Check sheet for the drawn part. Datum: minimum x, y, z corner. Units: mm. A direction names the side the tool comes from. Give positions to 0.01 mm unless a question says otherwise; leave off trailing zeros. Loops run counter-clockwise (first coordinate to the right, second up) from the corner with the lowest first, then second, coordinate; pieces in that order, holes last. Notation, with made-up numbers: (64.25, -12.5) - (89.25, -12.5) arc R10 ccw to (89.25, 2.5) - close; hole circle Ø5 at (-14, 44). An arc over 180 degrees is marked (long way). One line per item, written item: value. Start each with the question number.
1. Scan lines: L1, parallel to X at y = 3.9, z = 4; L2, parallel to Y at x = 10.75, z = 7; L3, parallel to Z at x = 8.75, y = 2.1. Record each from-to range of solid material in increasing order. Write a range as [from, to].
2. Sectioned sample at D-D (y = 1.65). Record the cut outline in (x, z), plus the area to 3 significant figures.
3. Sectioned sample at B-B (x = 7). Record the cut outline in (y, z), plus the area to 3 significant figures.
4. Sectioned sample at C-C (z = 4). Record the cut outline in (x, y).
5. Access from +Z, -Z, +X, -X, +Y, -Y to the whole of each face (thin tool, end or side, straight path). Record for the marked faces 1, 2, 3, 4 and 5.
6. Mould release check, pull along X, two halves, no side actions. Record for the marked faces 6, 7, 8 and 9: pulls with the +X half, pulls with the -X half, needs draft (parallel to the pull), parting line crosses it, or undercut.
7. Sectioned sample at A-A (y = 3). Record the cut outline in (x, z).
8. Gauge pin test, flat ends, axial feed: pin 1 (0.8 mm diameter, centred on y = 1.5, z = 4.5, fed in from -X); pin 2 (2 mm diameter, centred on x = 7, z = 4.5, fed in from +Y); pin 3 (2 mm diameter, centred on x = 6.5, y = 1, fed in from -Z); pin 4 (1 mm diameter, centred on y = 2.5, z = 2.5, fed in from -X). Record the tip position at first contact, or that the pin passes through.
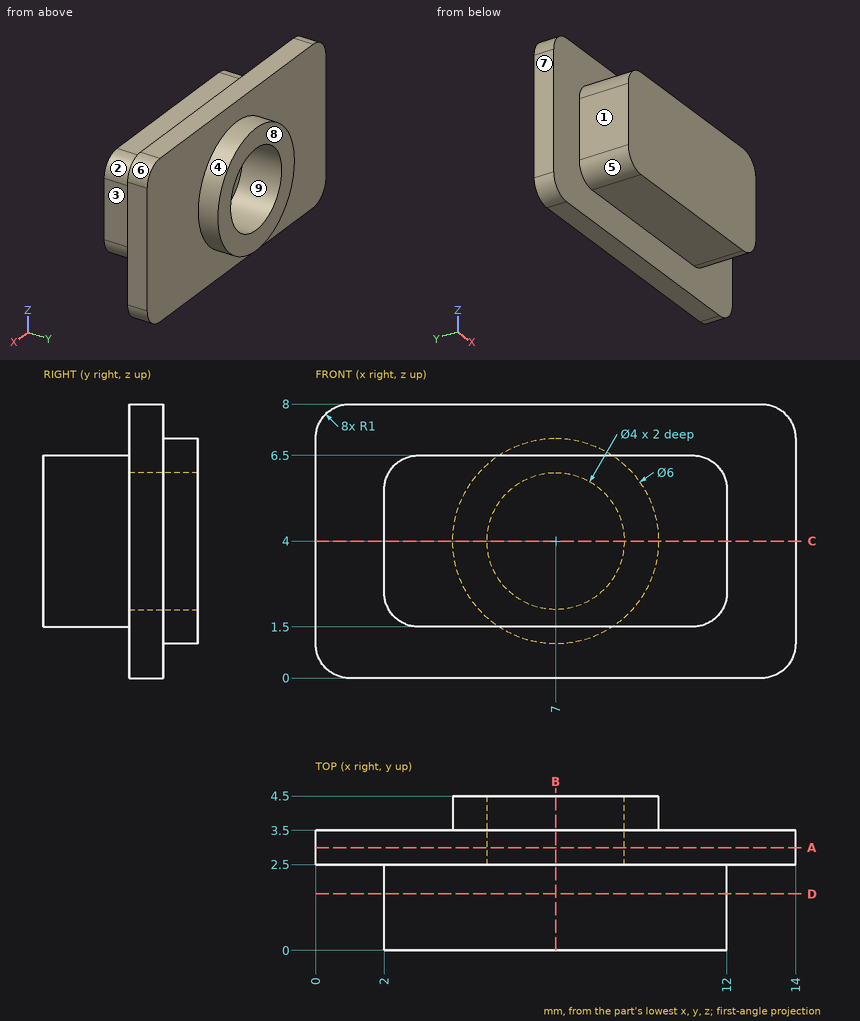
Results are:
1. L1: x = [4, 5], [9, 10]
1. L2: y = [2.5, 3.5]
1. L3: z = [1.5, 6.5]
2. outline: (2, 2.5) arc R1 ccw to (3, 1.5) - (11, 1.5) arc R1 ccw to (12, 2.5) - (12, 5.5) arc R1 ccw to (11, 6.5) - (3, 6.5) arc R1 ccw to (2, 5.5) - close
2. area: 49.1 mm^2
3. outline: (0, 1.5) - (2.5, 1.5) - (2.5, 0) - (3.5, 0) - (3.5, 1) - (4.5, 1) - (4.5, 2) - (2.5, 2) - (2.5, 6) - (4.5, 6) - (4.5, 7) - (3.5, 7) - (3.5, 8) - (2.5, 8) - (2.5, 6.5) - (0, 6.5) - close
3. area: 18.5 mm^2
4. outline: (0, 2.5) - (2, 2.5) - (2, 0) - (12, 0) - (12, 2.5) - (14, 2.5) - (14, 3.5) - (10, 3.5) - (10, 4.5) - (9, 4.5) - (9, 2.5) - (5, 2.5) - (5, 4.5) - (4, 4.5) - (4, 3.5) - (0, 3.5) - close
5. face 1: +Z, -Z, -X, -Y
5. face 2: +Z, +X, -Y
5. face 3: +Z, -Z, +X, -Y
5. face 4: +Y
5. face 5: -Z, -X, -Y
6. face 6: pulls with the +X half
6. face 7: pulls with the -X half
6. face 8: needs draft
6. face 9: undercut
7. outline: (0, 1) arc R1 ccw to (1, 0) - (13, 0) arc R1 ccw to (14, 1) - (14, 7) arc R1 ccw to (13, 8) - (1, 8) arc R1 ccw to (0, 7) - close; hole circle Ø4 at (7, 4)
8. pin 1: stops at x = 2
8. pin 2: stops at y = 2.5
8. pin 3: stops at z = 1.5
8. pin 4: stops at x = 0
